Autodesk Inventor part; units mm, degrees
ref_plane "YZ Plane" through (0, 0, 0) normal (1, 0, 0) x (0, 1, 0)
ref_plane "XZ Plane" through (0, 0, 0) normal (0, 1, 0) x (-1, 0, 0)
ref_plane "XY Plane" through (0, 0, 0) normal (0, 0, 1) x (1, 0, 0)
sketch "Sketch1" plane through (0, 0, 0) normal (0, 0, 1) x (1, 0, 0)
  line L0 (-134, -47.5) -> (134, -47.5)
  line L1 (134, -47.5) -> (134, 47.5)
  line L2 (134, 47.5) -> (-134, 47.5)
  line L3 (-134, 47.5) -> (-134, -47.5)
  line L4 (-134, -47.5) -> (134, 47.5) construction
  line L5 (134, -47.5) -> (-134, 47.5) construction
  point P0 (0, 0)
  dimension "d0" = 95
  dimension "d1" = 268
extrude "Extrusion1" add sketch "Sketch1" along normal blind 6
sketch "Sketch2" plane through (0, 0, 6) normal (0, 0, 1) x (1, 0, 0)
  line L0 (-134, 47.5) -> (-134, -47.5)
  line L1 (-131.125, -39.5) -> (-124.875, -39.5)
  line L2 (-124.875, -39.5) -> (-124.875, 39.5)
  line L3 (-124.875, 39.5) -> (-131.125, 39.5)
  line L4 (-131.125, 39.5) -> (-131.125, -39.5)
  line L5 (-131.125, -39.5) -> (-124.875, 39.5) construction
  line L6 (-124.875, -39.5) -> (-131.125, 39.5) construction
  line L7 (124.875, -39.5) -> (131.125, -39.5)
  line L8 (131.125, -39.5) -> (131.125, 39.5)
  line L9 (131.125, 39.5) -> (124.875, 39.5)
  line L10 (124.875, 39.5) -> (124.875, -39.5)
  line L11 (124.875, -39.5) -> (131.125, 39.5) construction
  line L12 (131.125, -39.5) -> (124.875, 39.5) construction
  line L13 (-134, -47.5) -> (134, -47.5)
  line L14 (134, -47.5) -> (134, 47.5)
  point P0 (0, 0)
  point P1 (-128, 0)
  point P2 (128, 0)
  dimension "d4" = 6.25
  dimension "d5" = 2.875
  dimension "d23" = 8
  dimension "d24" = 2.875
extrude "Extrusion2" cut sketch "Sketch2" against normal through all
fillet "Fillet2" radius 3 2 edges at (-134, -47.5, 3) (134, -47.5, 3)
sketch "Sketch3" plane through (0, 0, 6) normal (0, 0, 1) x (1, 0, 0)
  line L0 (134, 47.5) -> (-134, 47.5)
  line L1 (-150, 47.5) -> (134, 47.5)
  line L2 (134, 47.5) -> (134, 72.5)
  line L3 (134, 72.5) -> (-150, 72.5)
  line L4 (-150, 72.5) -> (-150, 47.5)
  point P0 (0, 0)
  dimension "d12" = 25
  dimension "d25" = 150
extrude "Extrusion3" add sketch "Sketch3" against normal blind 6
fillet "Fillet3" radius 3 4 edges at (134, 72.5, 3) (-150, 47.5, 3) (-150, 72.5, 3) (-134, 47.5, 3)
sketch "Sketch5" plane through (0, 0, 6) normal (0, 0, 1) x (1, 0, 0)
  line L0 (-150, 50.5) -> (-150, 69.5)
  line L1 (-147, 72.5) -> (131, 72.5)
  circle A0 centre (-77.306, 53.053) radius 2.286
  circle A1 centre (-45.556, 53.053) radius 2.286
  point P0 (0, 0)
  dimension "d26" = 72.694
  dimension "d27" = 31.75
  dimension "d28" = 19.447
  dimension "d29" = 4.572
extrude "Extrusion5" cut sketch "Sketch5" against normal blind 10
equation "\"d24\" = d5"
properties part number "TopTopPanel"
The listing builds one solid part. Answer for the finished solid, in the listing's coordinates (mm). A direction names the side the tool comes from. Coordinates: 2 decimals unless noted, no trailing zeros. Write each loop counter-clockwise with the first axis right and the second up, starting at its lowest first coordinate (ties: lowest second). Pieces come first, ordered by that corner, then holes.
Q1. Given P1, Ø3.5, axis at x = -45.556, y = 53.053, coming from the +Z side, flat-ended and moving along its own axis, determine where the tip first touches the part or whether it passes through.
Returned:
P1: passes through
Q2. Which of the six approach directions +Z, -Z, +X, -X, +Y, -Y give full straight-line access (tool end or side, diameter ignored) to faces 1 (the flat face through (-2, -47.5, 3)), 2 (the flat face through (124.875, 1, 3)), 3 (the flat face through (-142, 47.5, 3))?
Returned:
face 1: +Z, -Z, +X, -X, -Y
face 2: +Z, -Z
face 3: +Z, -Z, -X, -Y
Q3. Section B-B, the plane z = 4.9 is taken. Write down the section's boundary in (x, y) (3 decimals).
Returned:
outline: (-150, 50.5) arc R3 ccw to (-147, 47.5) - (-137, 47.5) arc R3 cw to (-134, 44.5) - (-134, -44.5) arc R3 ccw to (-131, -47.5) - (131, -47.5) arc R3 ccw to (134, -44.5) - (134, 69.5) arc R3 ccw to (131, 72.5) - (-147, 72.5) arc R3 ccw to (-150, 69.5) - close; hole (-131.125, -39.5) - (-124.875, -39.5) - (-124.875, 39.5) - (-131.125, 39.5) - close; hole circle Ø4.572 at (-77.306, 53.053); hole circle Ø4.572 at (-45.556, 53.053); hole (124.875, -39.5) - (131.125, -39.5) - (131.125, 39.5) - (124.875, 39.5) - close
Q4. The mould has two halves that part along X. Classify faces 4 (the flat face through (-150, 60, 3)), 5 (the flat face through (-131.125, 1, 3)), 6 (the flat face through (-10, 13, 6)), 7 (the flat face through (134, 12, 3)): released by +X, released by -X, zero draft, split by the parting line, or undercut.
Returned:
face 4: released by -X
face 5: undercut
face 6: zero draft
face 7: released by +X
Q5. Find the intervals of material crossed by line 1 along X through (y, z) = (-27, 0.75) (3 decimals); line 2 along X through (y, z) = (-40.5, 3.45); line 3 along X through (y, z) = (50, 4.65), in increasing order.
Returned:
line 1: x = -134 to -131.125, -124.875 to 124.875, 131.125 to 134
line 2: x = -134 to 134
line 3: x = -149.96 to 134
Q6. Section A-A, the plane y = -24.5 is taken. Write down the section's boundary in (x, z) (3 decimals).
Returned:
outline: (-134, 0) - (-131.125, 0) - (-131.125, 6) - (-134, 6) - close; (-124.875, 0) - (124.875, 0) - (124.875, 6) - (-124.875, 6) - close; (131.125, 0) - (134, 0) - (134, 6) - (131.125, 6) - close
